from build123d import *

# Parameters (mm, degrees)
SKETCH1_W               = 37
SKETCH1_H               = 58
BOSS_EXTRUDE1_DEPTH     = 30
SKETCH2_W               = 33
SKETCH2_H               = 13
CUT_EXTRUDE1_DEPTH      = 54
CUT_EXTRUDE2_DEPTH      = 46
M4_CLEARANCE_HOLE1_D    = 4.3
M4_CLEARANCE_HOLE2_D    = 4.3
SKETCH8_W               = 37
SKETCH8_H               = 13
CUT_EXTRUDE3_DEPTH      = 55
CUT_EXTRUDE3_DEPTH_BACK = 10
FILLET1_R               = 0.5
BOSS_EXTRUDE2_DEPTH     = 2


with BuildPart() as part:
    # Sketch1 → Boss-Extrude1 (new body)
    with BuildSketch(Plane.XY):
        with Locations((18.5, 29)):
            Rectangle(SKETCH1_W, SKETCH1_H)
    extrude(amount=BOSS_EXTRUDE1_DEPTH)

    # Sketch2 → Cut-Extrude1 (cut)
    with BuildSketch(Plane(origin=(0, 58, 0), x_dir=(1, 0, 0), z_dir=(0, 1, 0))):
        with Locations((20.5, -6.5)):
            Rectangle(SKETCH2_W, SKETCH2_H)
        with Locations((20.5, -23.5)):
            Rectangle(SKETCH2_W, SKETCH2_H)
    extrude(amount=-CUT_EXTRUDE1_DEPTH, mode=Mode.SUBTRACT)

    # Sketch3 → Cut-Extrude2 (cut)
    with BuildSketch(Plane.XY.offset(13)):
        Polygon((4, 58), (37, 4), (37, 58), align=None)
    extrude(amount=CUT_EXTRUDE2_DEPTH, mode=Mode.SUBTRACT)

    # M4 Clearance Hole1 (through all)
    with Locations(Plane(origin=(4, 0, 0), x_dir=(0, 0, -1), z_dir=(1, 0, 0))):
        with Locations((-26.5, 14), (-26.5, 50)):
            Hole(M4_CLEARANCE_HOLE1_D / 2)

    # M4 Clearance Hole2 (through all)
    with Locations(Plane(origin=(0, 4, 0), x_dir=(1, 0, 0), z_dir=(0, 1, 0))):
        with Locations((12, -26.5), (30, -26.5)):
            Hole(M4_CLEARANCE_HOLE2_D / 2)

    # Sketch8 → Cut-Extrude3 (cut, two sides)
    with BuildSketch(Plane(origin=(0, 4, 0), x_dir=(1, 0, 0), z_dir=(0, 1, 0))) as cut_extrude3_sk:
        with Locations((18.5, -6.5)):
            Rectangle(SKETCH8_W, SKETCH8_H)
    extrude(amount=CUT_EXTRUDE3_DEPTH, mode=Mode.SUBTRACT)
    extrude(cut_extrude3_sk.sketch, amount=-CUT_EXTRUDE3_DEPTH_BACK, mode=Mode.SUBTRACT)

    # Fillet1
    fillet1_edges = [part.edges().sort_by_distance(p)[0] for p in [
        (4, 31, 17),
        (0, 29, 13),
    ]]
    fillet(fillet1_edges, radius=FILLET1_R)

    # Sketch9 → Boss-Extrude2 (add)
    with BuildSketch(Plane.XY.offset(30)):
        Polygon((0, 58), (4, 58), (4, 4), (37, 4), (37, 0), (0, 0), align=None)
    extrude(amount=BOSS_EXTRUDE2_DEPTH)


solid = part.part
The listing builds one solid part. Answer for the finished solid, in the listing's coordinates (mm). A direction names the side the tool comes from. Give positions to 0.01 mm unless a question says otherwise; leave off trailing zeros. Write each loop counter-clockwise with the first axis right and the second up, starting at its lowest first coordinate (ties: lowest second). Pieces come first, ordered by that corner, then holes.
1) Given P1, Ø6, axis at y = 25.5, z = 27, coming from the +X side; P2, Ø7.5, axis at x = 16.5, z = 28, coming from the +Y side; P3, Ø6, axis at x = 32.5, y = 14.5, coming from the +Z side, each flat-ended and moving along its own axis, determine where each tip first touches the part or whether it passes through.
2) Section B-B (y = 14) is taken. Write down the section's boundary in (x, z), and give its area (3 significant figures).
3) A tool of negligible diameter and unlimited length cuts with its end or side. For faces 1 (the face through (13, 19, 17)), 2 (the face through (37, 2, 22)), from which of +Z, -Z, +X, -X, +Y, -Y can it reach the whole face along a straight path? Write none if from no direction.
4) Find the intervals of material crossed by L1, parallel to X at y = 2.4, z = 26.5; L2, parallel to Y at x = 1.2, z = 26.5; L3, parallel to Z at x = 30, y = 2.4, in increasing order.
5) Section A-A (z = 26.5) is taken. Write down the section's boundary in (x, y).
6) Section C-C (x = 11) is taken. Write down the section's boundary in (y, z), and give its area (3 significant figures).
7) Section D-D (x = 34.5) is taken. Write down the section's boundary in (y, z).
8) For a pull along X with two mould halves and no side action, classify faces 3 (the face through (1.97, 51.81, 27.66)), 4 (the face through (4, 31, 25)), 5 (the face through (11.01, 1.97, 28.41)) as pulls with the +X half, pulls with the -X half, needs draft (parallel to the pull), parting line crosses it, or undercut.
Response:
1. P1: stops at x = 4
1. P2: stops at y = 4
1. P3: stops at z = 17
2. outline: (0, 13.5) arc R0.5 ccw to (0.5, 13) - (30.89, 13) - (30.89, 17) - (4.5, 17) arc R0.5 cw to (4, 17.5) - (4, 24.35) - (0, 24.35) - close; (0, 28.65) - (4, 28.65) - (4, 32) - (0, 32) - close
2. area: 166 mm2
3. face 1: +Z, +X, +Y
3. face 2: +Z, -Z, +X, +Y, -Y
4. L1: x = 0 to 9.85, 14.15 to 27.85, 32.15 to 37
4. L2: y = 0 to 11.85, 16.15 to 47.85, 52.15 to 58
4. L3: z = 13 to 24.35, 28.65 to 32
5. outline: (0, 0) - (9.85, 0) - (9.85, 4) - (4, 4) - (4, 11.85) - (0, 11.85) - close; (0, 16.15) - (4, 16.15) - (4, 47.85) - (0, 47.85) - close; (0, 52.15) - (4, 52.15) - (4, 58) - (0, 58) - close; (14.15, 0) - (27.85, 0) - (27.85, 4) - (14.15, 4) - close; (32.15, 0) - (37, 0) - (37, 4) - (32.15, 4) - close
6. outline: (0, 13) - (46.55, 13) - (46.55, 17) - (4, 17) - (4, 24.6) - (0, 24.6) - close; (0, 28.4) - (4, 28.4) - (4, 32) - (0, 32) - close
6. area: 231 mm2
7. outline: (0, 13) - (8.09, 13) - (8.09, 17) - (4, 17) - (4, 32) - (0, 32) - close
8. face 3: needs draft
8. face 4: pulls with the +X half
8. face 5: undercut
